from build123d import *

# Parameters (mm, degrees)
PERIMETER_START     = -6.19
PERIMETER_DEPTH     = 8.19
FILLET1_R           = 3
BOSS_EXTRUDE3_START = 2
SKETCH2_8_W         = 5.473282091
SKETCH2_8_H         = 4.239040608
BOSS_EXTRUDE3_DEPTH = 2
FILLET3_R           = 3


with BuildPart() as part:
    # Sketch2 → Perimeter (new body)
    with BuildSketch(Plane.XY.offset(PERIMETER_START)):
        Polygon((131.091872, -113.860488221), (131.091872, -125.165005986), (164.307694987, -125.165005986), (164.307694987, -114.861877626), (164.307694987, -107.096275934), (164.307694987, -98.754254601), (131.091872, -98.754254601), (131.091872, -106.09488653), align=None)
        Polygon((133.091872, -99.55), (152.68714679, -99.55), (156.626717909, -99.55), (162.307694987, -99.55), (162.307694987, -123.165005986), (133.091872, -123.165005986), align=None, mode=Mode.SUBTRACT)
    extrude(amount=PERIMETER_DEPTH)

    # Fillet1
    fillet1_edges = [part.edges().sort_by_distance(p)[0] for p in [
        (133.091872, -123.165005986, -2.095),
        (131.091872, -125.165005986, -2.095),
    ]]
    fillet(fillet1_edges, radius=FILLET1_R)

    # Sketch2<8> → Boss-Extrude3 (add)
    # profile 1 of 2: a face of its own
    with BuildSketch(Plane.XY.offset(BOSS_EXTRUDE3_START)):
        Polygon((131.091872, -113.860488221), (131.091872, -125.165005986), (164.307694987, -125.165005986), (164.307694987, -114.861877626), (164.307694987, -107.096275934), (164.307694987, -98.754254601), (131.091872, -98.754254601), (131.091872, -106.09488653), align=None)
        Polygon((133.091872, -99.55), (152.68714679, -99.55), (156.626717909, -99.55), (162.307694987, -99.55), (162.307694987, -123.165005986), (133.091872, -123.165005986), align=None, mode=Mode.SUBTRACT)
    # profile 2 of 2: a face of its own
    with BuildSketch(Plane.XY.offset(BOSS_EXTRUDE3_START)):
        Polygon((156.626717909, -102.601169367), (152.68714679, -102.601169367), (152.68714679, -99.55), (133.091872, -99.55), (133.091872, -123.165005986), (162.307694987, -123.165005986), (162.307694987, -99.55), (156.626717909, -99.55), align=None)
        with Locations((159.363358955, -116.030479696)):
            Rectangle(SKETCH2_8_W, SKETCH2_8_H, mode=Mode.SUBTRACT)
    extrude(amount=BOSS_EXTRUDE3_DEPTH)

    # Fillet3
    fillet3_edges = [part.edges().sort_by_distance(p)[0] for p in [
        (131.091872, -125.165005986, 3),
    ]]
    fillet(fillet3_edges, radius=FILLET3_R)


solid = part.part
For this review, take the finished solid that the model builds, in its own axes (mm). A direction names the side the tool comes from. Round coordinates to 2 decimals unless told otherwise and drop trailing zeros. Write each loop counter-clockwise with the first axis right and the second up, starting at its lowest first coordinate (ties: lowest second). Pieces come first, ordered by that corner, then holes. Notation, with made-up numbers: (-30, -17) - (17, -17) arc R25 cw to (17, 15) - close; hole circle Ø4 at (-25.75, 52). An arc over 180 degrees is marked (long way). Write item = value, one per line. Start each with the question number.
1. Consider section C-C on y = -117.5. State the section outline as (x, z) points.
2. Consider section A-A on x = 161.5. State the section outline as (y, z) points (3 decimals), plus the area to 3 significant figures.
3. Wall thickness on L1, parallel to Y at x = 153, z = -1.75 (3 decimals); L2, parallel to X at y = -111, z = 1; L3, parallel to X at y = -115.75, z = 2.75: over which ranges is each line inside the solid? List them lowest first.
4. For pin 1 Ø1 at (x, y) = (147, -101.5) entering from -Z, flat-tipped, find the tip position at first contact; note if it passes through.
5. Consider section D-D on z = -0.75. State the section outline as (x, y) points (3 decimals), plus the area to 3 significant figures.
6. Draft analysis for pull direction X (two halves, no side actions). For faces 4 (the face through (148, -98.754, -1)), 5 (the face through (164.308, -112, -1)), 6 (the face through (159, -113.911, 3)), state which applies: released by +X, released by -X, zero draft, split by the parting line, or undercut.
7. For faces 1 (the face through (133.947, -122.263, -2.038)), 2 (the face through (162.1, -116, 3)), 3 (the face through (148, -124, -6.19)), list the 3-axis set-ups (+Z, -Z, +X, -X, +Y, -Y) from which the entire face can be reached by the end or side of a thin tool; tool diameter is ignored.
8. Consider section B-B on z = 2.5. State the section outline as (x, y) points (3 decimals).
Evaluation:
q1.outline = (131.09, -6.19) - (133.09, -6.19) - (133.09, 2) - (156.63, 2) - (156.63, 4) - (131.09, 4) - close; (162.1, 2) - (162.31, 2) - (162.31, -6.19) - (164.31, -6.19) - (164.31, 4) - (162.1, 4) - close
q2.outline = (-125.165, -6.19) - (-123.165, -6.19) - (-123.165, 2) - (-118.15, 2) - (-118.15, 4) - (-125.165, 4) - close; (-113.911, 2) - (-99.55, 2) - (-99.55, -6.19) - (-98.754, -6.19) - (-98.754, 4) - (-113.911, 4) - close
q2.area = 67.2 mm2
q3.L1 = -125.165 to -123.165, -99.55 to -98.754
q3.L2 = 131.09 to 133.09, 162.31 to 164.31
q3.L3 = 131.09 to 156.63, 162.1 to 164.31
q4.pin_1 = 2
q5.outline = (131.092, -122.165) arc R3 ccw to (134.092, -125.165) - (164.308, -125.165) - (164.308, -98.754) - (131.092, -98.754) - close; hole (133.092, -120.165) arc R3 ccw to (136.092, -123.165) - (162.308, -123.165) - (162.308, -99.55) - (133.092, -99.55) - close
q5.area = 187 mm2
q6.face_4 = zero draft
q6.face_5 = released by +X
q6.face_6 = undercut
q7.face_1 = -Z
q7.face_2 = +Z, -Z
q7.face_3 = -Z, +X, -X, +Y, -Y
q8.outline = (131.092, -122.165) arc R3 ccw to (134.092, -125.165) - (164.308, -125.165) - (164.308, -98.754) - (131.092, -98.754) - close; hole (152.687, -102.601) - (156.627, -102.601) - (156.627, -99.55) - (152.687, -99.55) - close; hole (156.627, -118.15) - (162.1, -118.15) - (162.1, -113.911) - (156.627, -113.911) - close
